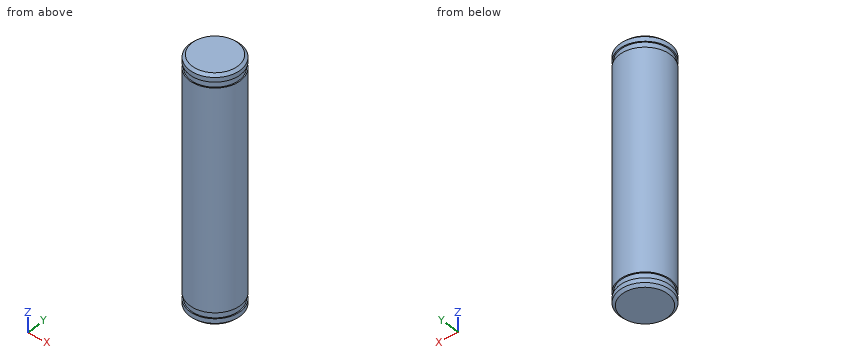
```python
from build123d import *

# Parameters (mm, degrees)
SKETCH1_W     = 60.325
SKETCH1_H     = 6.223
SKETCH2_W     = 1.4224
SKETCH2_H     = 0.8128
CHAMFER1_SIZE = 0.635


with BuildPart() as part:
    # Sketch1 → Revolve1 (revolve)
    with BuildSketch(Plane(origin=(0, 0, 0), x_dir=(0, 0, -1), z_dir=(1, 0, 0)), mode=Mode.PRIVATE) as revolve1_sk:
        with Locations((30.1625, 3.1115)):
            Rectangle(SKETCH1_W, SKETCH1_H)
    revolve(revolve1_sk.sketch.rotate(Axis((0, 0, 0), (0, 0, 1)), 90), axis=Axis((0, 0, 0), (0, 0, 1)))

    # Sketch2 → Cut-Revolve1 (revolve, cut)
    with BuildSketch(Plane(origin=(0, 0, 0), x_dir=(0, 0, -1), z_dir=(1, 0, 0)), mode=Mode.PRIVATE) as cut_revolve1_sk:
        with Locations((2.4638, 6.35)):
            Rectangle(SKETCH2_W, SKETCH2_H)
        with Locations((57.8612, 6.35)):
            Rectangle(SKETCH2_W, SKETCH2_H)
    revolve(cut_revolve1_sk.sketch.rotate(Axis((0, 0, 0), (0, 0, 1)), 90), axis=Axis((0, 0, 0), (0, 0, 1)), mode=Mode.SUBTRACT)

    # Chamfer1
    chamfer1_edges = [part.edges().sort_by_distance(p)[0] for p in [
        (6.223, 0, -60.325),
        (6.223, 0, 0),
    ]]
    chamfer(chamfer1_edges, length=CHAMFER1_SIZE)


solid = part.part
```
Model file for the job. Use its own axes, mm. Round coordinates to 2 decimals unless told otherwise and drop trailing zeros. Order: outer loops, then holes, each group sorted by start corner. A loop starts at its lowest first (then second) coordinate and runs counter-clockwise, first axis right, second up. Notation, with made-up numbers: M 75,32 L 134,32 A28 ccw 134,56 Z; hole C 36,12.5 d11. An arc over 180 degrees is marked long. Use CSV: the item, a comma, the result in double quotes.
Item 1: Saw through at A-A (z = -32.5). List the corners of the cut face in (x, y), plus the area to 3 significant figures.
Worked answers:
outline,"C 0,0 d12.45"
area,"122 mm²"
Item 2: Pin check, flat tips, straight feed: pin 1 (1 mm diameter, centred on x = 2.5, z = -26.5, fed in from -Y); pin 2 (5 mm diameter, centred on y = -5, z = -20, fed in from +X); pin 3 (1 mm diameter, centred on y = 1.5, z = -7.5, fed in from -X). Stop position of each tip, or through.
Worked answers:
pin 1,"y = -5.89"
pin 2,"x = 5.7"
pin 3,"x = -6.14"
Item 3: Probe probe 1 along X at (y, z) = (0.25, -47); probe 2 along X at (y, z) = (-2.75, -33.5). List the from-to ranges inside material, lowest first.
Worked answers:
probe 1,"-6.22 to 6.22"
probe 2,"-5.58 to 5.58"
